Source: CAD feature listing. Evaluate the final solid. Frame: model axes, mm. Face numbers are marked on the shaded views. A direction names the side the tool comes from. Give positions to 0.01 mm unless a question says otherwise; leave off trailing zeros. Order: outer loops, then holes, each group sorted by start corner. A loop starts at its lowest first (then second) coordinate and runs counter-clockwise, first axis right, second up.
```python
from build123d import *
from OCP.BRepFilletAPI import BRepFilletAPI_MakeChamfer

# Parameters (mm, degrees)
BOSS_EXTRUDE1_DEPTH     = 40
CUT_EXTRUDE1_DEPTH      = 30
CUT_EXTRUDE1_DEPTH_BACK = 30
CHAMFER1_SIZE           = 2
CHAMFER1_SIZE2          = 1.538618516
CHAMFER1_SIZE2_2        = 2.126587288
SKETCH3_R               = 1.6
CUT_EXTRUDE2_DEPTH      = 10
SKETCH4_W               = 6
SKETCH4_H               = 8.2
BOSS_EXTRUDE2_DEPTH     = 12
CHAMFER2_SIZE           = 3
CHAMFER3_SIZE           = 0.8
CUT_EXTRUDE3_DEPTH      = 47.848799344
CUT_EXTRUDE3_DEPTH_BACK = 47.848799344
SKETCH5_R               = 1.625
RIB1_REACH              = 43.809
SKETCH8_WALL_W          = 116.212296924
SKETCH8_WALL_H          = 2


with BuildPart() as part:
    # Sketch1 → Boss-Extrude1 (new body)
    with BuildSketch(Plane.XY):
        Polygon((0, 0), (12, 0), (0, -30), (18, -30), (18, -32), (-2.954065923, -32), (9.045934077, -2), (0, -2), align=None)
    extrude(amount=BOSS_EXTRUDE1_DEPTH)

    # Sketch2 → Cut-Extrude1 (cut, two sides: drawn at the far end of the back side and taken through both)
    with BuildSketch(Plane.ZY.offset(-CUT_EXTRUDE1_DEPTH_BACK)):
        Polygon((15.099668871, -16), (1.887458609, -2), (0, -2), (0, -32), align=None)
        Polygon((40, -2), (38.112541391, -2), (24.900331129, -16), (40, -32), align=None)
    extrude(amount=CUT_EXTRUDE1_DEPTH + CUT_EXTRUDE1_DEPTH_BACK, mode=Mode.SUBTRACT)

    # Chamfer1: one chamfer whose edges measure the first distance from different faces: ONE call of the kernel's chamfer builder (chamfer() names one face for all edges)
    chamfer1_edges_1 = [part.edges().sort_by_distance(p)[0] for p in [
        (0, -30, 20),
    ]]
    chamfer1_side_1 = [part.faces().sort_by_distance(p)[0] for p in [
        (9, -30, 20),
    ]]
    chamfer1_edges_2 = [part.edges().sort_by_distance(p)[0] for p in [
        (9.045934077, -2, 20),
    ]]
    chamfer1_side_2 = [part.faces().sort_by_distance(p)[0] for p in [
        (4.646047571, -2, 20),
    ]]
    chamfer1_edges_3 = [part.edges().sort_by_distance(p)[0] for p in [
        (4.522967039, -16, 24.900331129),
    ]]
    chamfer1_side_3 = [part.faces().sort_by_distance(p)[0] for p in [
        (7.322967039, -9, 31.50643626),
    ]]
    chamfer1_edges_4 = [part.edges().sort_by_distance(p)[0] for p in [
        (4.522967039, -16, 15.099668871),
    ]]
    chamfer1_side_4 = [part.faces().sort_by_distance(p)[0] for p in [
        (7.322967039, -9, 8.49356374),
    ]]
    chamfer1 = BRepFilletAPI_MakeChamfer(part.part.solid().wrapped)
    for e in chamfer1_edges_1:
        chamfer1.Add(CHAMFER1_SIZE, CHAMFER1_SIZE2, e.wrapped, chamfer1_side_1[0].wrapped)  # the first distance lies on this face
    for e in chamfer1_edges_2:
        chamfer1.Add(CHAMFER1_SIZE, CHAMFER1_SIZE2, e.wrapped, chamfer1_side_2[0].wrapped)  # the first distance lies on this face
    for e in chamfer1_edges_3:
        chamfer1.Add(CHAMFER1_SIZE, CHAMFER1_SIZE2_2, e.wrapped, chamfer1_side_3[0].wrapped)  # the first distance lies on this face
    for e in chamfer1_edges_4:
        chamfer1.Add(CHAMFER1_SIZE, CHAMFER1_SIZE2_2, e.wrapped, chamfer1_side_4[0].wrapped)  # the first distance lies on this face
    add(Compound.cast(chamfer1.Shape()), mode=Mode.REPLACE)

    # Sketch3 → Cut-Extrude2 (cut)
    with BuildSketch(Plane.XZ.offset(32)):
        Polygon((18, 40), (15, 40), (18, 28), align=None)
        Polygon((18, 0), (18, 12), (15, 0), align=None)
        with Locations(Location((12, 37, 0), (0, 0, 270))):
            Circle(SKETCH3_R)
        with Locations(Location((12, 3, 0), (0, 0, 270))):
            Circle(SKETCH3_R)
    extrude(amount=-CUT_EXTRUDE2_DEPTH, mode=Mode.SUBTRACT)

    # Sketch4 → Boss-Extrude2 (add)
    with BuildSketch(Plane.ZY):
        with Locations((13.9, 4.1)):
            Rectangle(SKETCH4_W, SKETCH4_H)
        with Locations((26.1, 4.1)):
            Rectangle(SKETCH4_W, SKETCH4_H)
    extrude(amount=-BOSS_EXTRUDE2_DEPTH)

    # Chamfer2
    chamfer2_edges = [part.edges().sort_by_distance(p)[0] for p in [
        (6, 0, 10.9),
        (6, 0, 29.1),
    ]]
    chamfer(chamfer2_edges, length=CHAMFER2_SIZE)

    # Chamfer3
    # the kernel refuses this chamfer: 0.8 mm, written as the material it adds along each edge
    with BuildSketch(Plane(origin=(0, 0, 16.9), x_dir=(0, 0.9996219169112966, -0.027495876610587354), z_dir=(1, 0, 0))) as chamfer3_piece_1_section:
        Polygon((CHAMFER3_SIZE * 0.999621916911, CHAMFER3_SIZE * 0.0274958766106), (-CHAMFER3_SIZE * 0.0274958766106, CHAMFER3_SIZE * 0.999621916911), (0, 0), align=None)
    chamfer3_piece_1 = extrude(amount=12, mode=Mode.PRIVATE)
    chamfer3_piece_1 = split(chamfer3_piece_1, bisect_by=Plane(origin=(11.263378783, -1.841553042, 17.163829715), z_dir=(-0.9284766908852594, 0.3713906763541038, 0)), keep=Keep.TOP, mode=Mode.PRIVATE)
    add(chamfer3_piece_1)
    with BuildSketch(Plane(origin=(0, 0, 23.1), x_dir=(0, 0.9996219169112966, 0.027495876610587354), z_dir=(1, 0, 0))) as chamfer3_piece_2_section:
        Polygon((CHAMFER3_SIZE * 0.999621916911, -CHAMFER3_SIZE * 0.0274958766106), (-CHAMFER3_SIZE * 0.0274958766106, -CHAMFER3_SIZE * 0.999621916911), (0, 0), align=None)
    chamfer3_piece_2 = extrude(amount=12, mode=Mode.PRIVATE)
    chamfer3_piece_2 = split(chamfer3_piece_2, bisect_by=Plane(origin=(11.263378783, -1.841553042, 22.836170285), z_dir=(-0.9284766908852594, 0.3713906763541038, 0)), keep=Keep.TOP, mode=Mode.PRIVATE)
    add(chamfer3_piece_2)
    # the kernel refuses this chamfer: 0.8 mm, written as the material it takes off along each edge
    with BuildSketch(Plane(origin=(-2.05734639, 8.2, 10.9), x_dir=(0, -0.9996219169112966, -0.02749587661058733), z_dir=(1, 0, 0)), Plane(origin=(-2.05734639, 8.2, 16.9), x_dir=(0, 0.027495876610587302, -0.9996219169112966), z_dir=(1, 0, 0)), Plane(origin=(-2.05734639, 8.2, 29.1), x_dir=(0, 0.027495876610587302, -0.9996219169112966), z_dir=(1, 0, 0)), Plane(origin=(-2.05734639, 8.2, 23.1), x_dir=(0, -0.9996219169112966, -0.02749587661058736), z_dir=(1, 0, 0))) as chamfer3_2_piece_1:
        Polygon((CHAMFER3_SIZE * 0.999621916911, -CHAMFER3_SIZE * 0.0274958766106), (-CHAMFER3_SIZE * 0.0274958766106, -CHAMFER3_SIZE * 0.999621916911), (0, 0), align=None)
    extrude(amount=16.114692781, mode=Mode.SUBTRACT)

    # Sketch5 → Cut-Extrude3 (cut, two sides: drawn at the far end of the back side and taken through both)
    with BuildSketch(Plane.XY.offset(29.1).offset(-CUT_EXTRUDE3_DEPTH_BACK)):
        with Locations(Location((6, 4.2, 0), (0, 0, 312.399473364))):
            Circle(SKETCH5_R)
    extrude(amount=CUT_EXTRUDE3_DEPTH + CUT_EXTRUDE3_DEPTH_BACK, mode=Mode.SUBTRACT)

    # Sketch8 wall → Rib1 (add, up to next)
    with BuildSketch(Plane(origin=(15, -15, 20), x_dir=(0.196116135138, -0.980580675691, 0), z_dir=(0.980580675691, 0.196116135138, 0)), mode=Mode.PRIVATE) as rib1_sk1:
        Rectangle(SKETCH8_WALL_W, SKETCH8_WALL_H)
    rib1_tool1 = extrude(rib1_sk1.sketch, amount=-RIB1_REACH, mode=Mode.PRIVATE) - part.part
    add(rib1_tool1.solids().sort_by_distance((15, -15, 20))[0])


solid = part.part
```
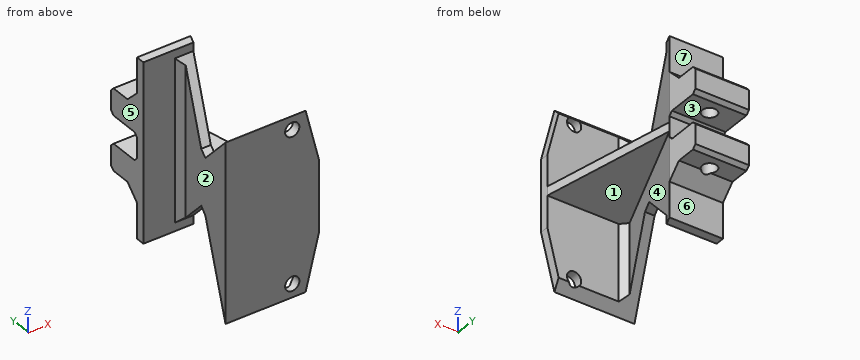
1) Section query D-D, the plane z = 19.5. Return the cut outline in (x, y), and give its area (3 significant figures).
Report:
outline: (-2.95, -32) - (18, -32) - (18, -30) - (12, 0) - (0, 0) - (0, -2) - (7.05, -2) - (8.47, -3.43) - close
area: 396 mm2
2) Material intervals for L1, parallel to X at y = 4.2, z = 25.75 (3 decimals); L2, parallel to Y at x = 4.75, z = 5; L3, parallel to Y at x = 2, z = 33, sorted ascending.
Report:
L1: x = 0 to 4.375, 7.625 to 12
L2: y = -32 to -30, -2 to 0
L3: y = -32 to -30, -25 to -24.58, -2 to 0
3) Draft query along Z for the marked faces 1, 2 and 3. Return one class per face: +Z half, -Z half, draft (parallel to the pull), parting line (faces both ways), or undercut.
Report:
face 1: -Z half
face 2: draft
face 3: undercut
4) Reachability of the marked faces 4, 5, 6 and 7 from +Z, -Z, +X, -X, +Y, -Y: full face, straight path, thin tool, end or side. Return the list, or none.
Report:
face 4: -Z, +X
face 5: +Z, -Z, -X, +Y
face 6: -Z, +X, -X, +Y
face 7: +Z, +X, -X, +Y
5) Section query B-B, the plane z = 27.5. Count the separate pieces of the cut face and the enclosed holes in it, and give its area (3 significant figures).
Report:
separate pieces: 2
enclosed holes: 1
area: 206 mm2
6) Pin query (flat end, axial travel): pin 1 (2 mm diameter, centred on x = 4.5, y = -23, fed in from +Z); pin 2 (8 mm diameter, centred on x = 1, y = -24.5, fed in from +Z); pin 3 (5 mm diameter, centred on x = 3.5, y = 4.5, fed in from +Z); pin 4 (2 mm diameter, centred on x = 6.5, y = 4.5, fed in from -Z). Return the tip coordinate at first contact, or that it passes through.
Report:
pin 1: stops at z = 21
pin 2: stops at z = 36.68
pin 3: stops at z = 30.1
pin 4: passes through
7) Section query A-A, the plane y = 4.2. Return the cut outline in (x, z) (3 decimals).
Report:
outline: (0, 10.9) - (4.375, 10.9) - (4.375, 16.9) - (0, 16.9) - close; (0, 23.1) - (4.375, 23.1) - (4.375, 29.1) - (0, 29.1) - close; (7.625, 10.9) - (12, 10.9) - (12, 16.9) - (7.625, 16.9) - close; (7.625, 23.1) - (12, 23.1) - (12, 29.1) - (7.625, 29.1) - close
